```python
from build123d import *

# Parameters (mm, degrees)
CROQUIS1_R              = 50.89009471
SALIENTE_EXTRUIR1_DEPTH = 150
CROQUIS2_R              = 17.571410618
CORTAR_EXTRUIR1_DEPTH   = 151
CROQUIS3_R              = 49.718427997
CROQUIS3_R_2            = 19.121829202
CORTAR_EXTRUIR2_DEPTH   = 2.5
CROQUIS4_R              = 19.476892412
CROQUIS4_R_2            = 17.829813716
SALIENTE_EXTRUIR3_DEPTH = 15
CROQUIS6_R              = 49.233249933
CROQUIS6_R_2            = 21.531739476
CORTAR_EXTRUIR4_DEPTH   = 5
CROQUIS8_W              = 2.81398907
CROQUIS8_H              = 5.576117682
SALIENTE_EXTRUIR6_DEPTH = 145
CROQUIS9_R              = 21.421140015
CROQUIS9_R_2            = 19.462987184
SALIENTE_EXTRUIR7_DEPTH = 2.5


with BuildPart() as part:
    # Croquis1 → Saliente-Extruir1 (new body)
    with BuildSketch(Plane(origin=(0, 0, 0), x_dir=(1, 0, 0), z_dir=(0, 1, 0))):
        Circle(CROQUIS1_R)
    extrude(amount=SALIENTE_EXTRUIR1_DEPTH)

    # Croquis2 → Cortar-Extruir1 (cut, through all)
    with BuildSketch(Plane(origin=(0, 150, 0), x_dir=(1, 0, 0), z_dir=(0, 1, 0))):
        Circle(CROQUIS2_R)
    extrude(amount=-CORTAR_EXTRUIR1_DEPTH, mode=Mode.SUBTRACT)

    # Croquis3 → Cortar-Extruir2 (cut)
    with BuildSketch(Plane(origin=(0, 150, 0), x_dir=(1, 0, 0), z_dir=(0, 1, 0))):
        Circle(CROQUIS3_R)
        Circle(CROQUIS3_R_2, mode=Mode.SUBTRACT)
    extrude(amount=-CORTAR_EXTRUIR2_DEPTH, mode=Mode.SUBTRACT)

    # Croquis4 → Saliente-Extruir3 (add)
    with BuildSketch(Plane.XZ):
        Circle(CROQUIS4_R)
        Circle(CROQUIS4_R_2, mode=Mode.SUBTRACT)
    extrude(amount=SALIENTE_EXTRUIR3_DEPTH)

    # Croquis6 → Cortar-Extruir4 (cut)
    with BuildSketch(Plane.XZ):
        Circle(CROQUIS6_R)
        Circle(CROQUIS6_R_2, mode=Mode.SUBTRACT)
    extrude(amount=-CORTAR_EXTRUIR4_DEPTH, mode=Mode.SUBTRACT)

    # Croquis8 → Saliente-Extruir6 (add)
    with BuildSketch(Plane(origin=(0, 147.5, 0), x_dir=(1, 0, 0), z_dir=(0, 1, 0))):
        with Locations((1.406994535, 14.783351777)):
            Rectangle(CROQUIS8_W, CROQUIS8_H)
        with Locations((1.406994535, -14.783351777)):
            Rectangle(CROQUIS8_W, CROQUIS8_H)
    extrude(amount=-SALIENTE_EXTRUIR6_DEPTH)

    # Croquis9 → Saliente-Extruir7 (add)
    with BuildSketch(Plane(origin=(0, 147.5, 0), x_dir=(1, 0, 0), z_dir=(0, 1, 0))):
        Circle(CROQUIS9_R)
        Circle(CROQUIS9_R_2, mode=Mode.SUBTRACT)
    extrude(amount=SALIENTE_EXTRUIR7_DEPTH)


solid = part.part
```
Input: part model. Units: mm. Frame: model coordinates. A direction names the side the tool comes from. Coordinates: 2 decimals unless noted, no trailing zeros. Write each loop counter-clockwise with the first axis right and the second up, starting at its lowest first coordinate (ties: lowest second). Pieces come first, ordered by that corner, then holes.
1) Pin query (flat end, axial travel): pin 1 Ø10 at (x, z) = (-33.5, -12) entering from -Y; pin 2 Ø1.5 at (x, z) = (-40.5, -22) entering from +Y; pin 3 Ø6 at (y, z) = (108.5, 16.5) entering from +X. Return the tip coordinate at first contact, or that it passes through.
2) Material intervals for line 1 along Z through (x, y) = (0, 148.15); line 2 along Z through (x, y) = (0, 1.4), sorted ascending.
3) Mould query, pull axis Z, two halves, no side actions, for faces 6 (the cylindrical face through (-14.36, -7.4, 13.16)), 7 (the flat face through (11, 150, 49)), 8 (the flat face through (21, 5, -10)). Classes: pulls with the +Z half, pulls with the -Z half, needs draft (parallel to the pull), parting line crosses it, or undercut.
4) Set-up query: faces 1 (the flat face through (0, 76, -15)), 2 (the cylindrical face through (-14.15, -7.4, -10.85)), 3 (the flat face through (5, 150, 19)), 4 (the cylindrical face through (20.432, 148.732, -6.434)), 5 (the flat face through (9, -15, -16)). Return all of +Z, -Z, +X, -X, +Y, -Y with unobstructed straight access to the full face (end or side cutting, diameter ignored); none if empty.
5) Section A-A on y = 80. Output: boundary loops of the cut face in (x, z).
Check result:
1. pin 1: stops at y = 5
1. pin 2: stops at y = 147.5
1. pin 3: stops at x = 49.07
2. line 1: z = -50.89 to -49.72, -21.42 to -19.46, -19.12 to -17.57, 17.57 to 19.12, 19.46 to 21.42, 49.72 to 50.89
2. line 2: z = -50.89 to -49.23, -21.53 to -17.57, 17.57 to 21.53, 49.23 to 50.89
3. face 6: parting line crosses it
3. face 7: needs draft
3. face 8: undercut
4. face 1: +Y, -Y
4. face 2: -Y
4. face 3: +Z, -Z, +X, -X, +Y
4. face 4: +Y
4. face 5: +Z, -Z, +X, -X, -Y
5. outline: circle Ø101.78 at (0, 0); hole (0, -17.57) - (0, -12) - (2.81, -12) - (2.81, -17.34) arc R17.57 ccw to (2.81, 17.34) - (2.81, 12) - (0, 12) - (0, 17.57) arc R17.57 ccw to start
